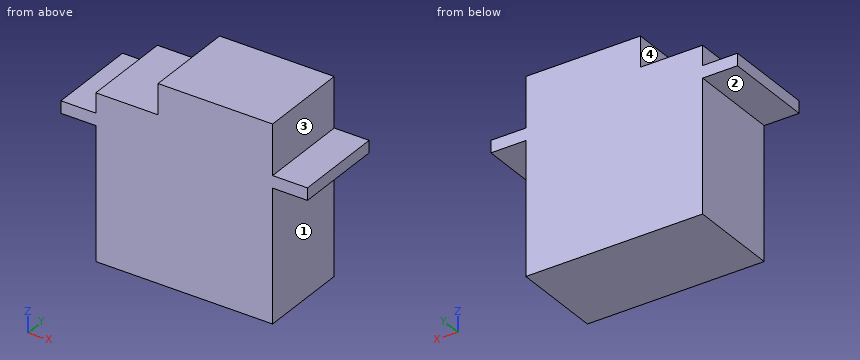
```python
from build123d import *

# Parameters (mm, degrees)
F0_W     = 23.3
F0_H     = 17.4
F0_W_2   = 15.1
F0_H_2   = 4
F0_H_3   = 1.6
F0_W_3   = 4.6
F1_DEPTH = 12


with BuildPart() as f1:
    # F0 (on Front) → F1 (new body)
    with BuildSketch(Plane.XZ):
        with Locations((11.65, -8.7)):
            Rectangle(F0_W, F0_H)
        with Locations((15.75, 6.2)):
            Rectangle(F0_W_2, F0_H_2)
        Polygon((8.2, 4.2), (0, 4.2), (0, 1.6), (23.3, 1.6), (23.3, 4.2), align=None)
        with Locations((11.65, 0.8)):
            Rectangle(F0_W, F0_H_3)
        with Locations((25.6, 0.8)):
            Rectangle(F0_W_3, F0_H_3)
        with Locations((-2.3, 0.8)):
            Rectangle(F0_W_3, F0_H_3)
    extrude(amount=F1_DEPTH)


solid = f1.part
```
Model file for the job. Use its own axes, mm. Face numbers are marked on the shaded views. A direction names the side the tool comes from. Give positions to 0.01 mm unless a question says otherwise; leave off trailing zeros. Write each loop counter-clockwise with the first axis right and the second up, starting at its lowest first coordinate (ties: lowest second). Pieces come first, ordered by that corner, then holes. Notation, with made-up numbers: (46.5, -2.75) - (56.5, -2.75) arc R25 ccw to (56.5, 28.25) - close; hole circle Ø5 at (10.5, -32.5). An arc over 180 degrees is marked (long way). One line per question, with ' | ' between items. Start each with the question number.
(1) 3-axis set-ups, long thin cutter, end or side, ignore diameter. For the marked faces 1, 2, 3 and 4: which of +Z, -Z, +X, -X, +Y, -Y reach the whole face in a straight line?
(2) Slice it at C-C on z = 4.75. Write the cut outline in (x, y).
(3) Pin check, flat tips, straight feed: P1, Ø2.5, axis at x = 4, y = -4, coming from the +Z side; P2, Ø3, axis at y = -6.5, z = 3.5, coming from the -X side; P3, Ø1.4, axis at x = -2, y = -6.5, coming from the +Z side. Stop position of each tip, or through.
(4) Wall check: line 1 along X through (y, z) = (-11, 6.25); line 2 along X through (y, z) = (-5, -11.75); line 3 along Z through (x, y) = (7, -7.5). Give the ranges that are in metal, low to high. Write a range as from..to.
(5) Slice it at A-A on y = -3.25. Write the cut outline in (x, z).
(6) Slice it at B-B on x = -1.5. Write the cut outline in (y, z), plus the area to 3 significant figures.
Results below:
1) face 1: -Z, +X, +Y, -Y | face 2: -Z, -X, +Y, -Y | face 3: +Z, +X, +Y, -Y | face 4: +Z, -X, +Y, -Y
2) outline: (8.2, -12) - (23.3, -12) - (23.3, 0) - (8.2, 0) - close
3) P1: z = 4.2 | P2: x = 0 | P3: z = 1.6
4) line 1: 8.2..23.3 | line 2: 0..23.3 | line 3: -17.4..4.2
5) outline: (-4.6, 0) - (0, 0) - (0, -17.4) - (23.3, -17.4) - (23.3, 0) - (27.9, 0) - (27.9, 1.6) - (23.3, 1.6) - (23.3, 8.2) - (8.2, 8.2) - (8.2, 4.2) - (0, 4.2) - (0, 1.6) - (-4.6, 1.6) - close
6) outline: (-12, 0) - (0, 0) - (0, 1.6) - (-12, 1.6) - close | area: 19.2 mm^2
